For this review, take the finished solid that the model builds, in its own axes (mm). A direction names the side the tool comes from. Round coordinates to 2 decimals unless told otherwise and drop trailing zeros. Answer in a Markdown table with one row per item. Add a question column.
from build123d import *

# Parameters (mm, degrees)
BOSS_EXTRUDE1_START = -2
SKETCH2_R           = 33.5
BOSS_EXTRUDE1_DEPTH = 2
SKETCH3_W           = 10
SKETCH3_H           = 15
CUT_EXTRUDE1_DEPTH  = 2


with BuildPart() as part:
    # Sketch1 → Revolve1 (revolve)
    with BuildSketch(Plane.XY, mode=Mode.PRIVATE) as revolve1_sk:
        with BuildLine():
            Line((-33.5, 0), (-33.5, 29))
            Line((-33.5, 29), (-35, 29))
            Line((-35, 29), (-35, 34))
            add(Edge.make_bspline(
                [(-35, 34), (-35, 84.230477341), (-10.204077545, 129), (0, 129)],
                knots=[0, 0, 0, 0, 1, 1, 1, 1], degree=3))
            Line((0, 129), (0, 128))
            add(Edge.make_bspline(
                [(-33.998483451, 34.678650605), (-33.991581263, 36.224092512), (-33.93035746, 39.323038638), (-33.628011861, 45.449717858), (-32.930147658, 52.999936547), (-31.637237127, 61.816356904), (-29.381428766, 73.174794828), (-25.705936414, 86.483124789), (-20.381782509, 100.569855924), (-15.566274854, 110.353659681), (-11.721562917, 116.772432581), (-8.903323702, 120.821784375), (-6.216251644, 124.044106905), (-4.149084944, 125.985259834), (-2.652724981, 127.059465204), (-1.628060193, 127.620483156), (-0.879863894, 127.88514238), (-0.348657385, 127.984548618), (-0.119526866, 128), (0, 128)],
                knots=[0.004535476, 0.004535476, 0.004535476, 0.004535476, 0.035643742, 0.066752009, 0.128968542, 0.191185074, 0.253401607, 0.377834673, 0.502267738, 0.626700804, 0.688917336, 0.751133869, 0.813350402, 0.875566935, 0.906675201, 0.937783467, 0.968891734, 0.984445867, 1, 1, 1, 1], degree=3))
            Line((-33.998483451, 34.678650605), (-34, 33.678651755))
            Line((-34, 33.678651755), (-34, 30))
            Line((-34, 30), (-32.5, 30))
            Line((-32.5, 30), (-32.5, 0))
            Line((-32.5, 0), (-33.5, 0))
        make_face()
    revolve(revolve1_sk.sketch.rotate(Axis((0, 0, 0), (0, 1, 0)), 270), axis=Axis((0, 0, 0), (0, 1, 0)))

    # Sketch2 → Boss-Extrude1 (add)
    with BuildSketch(Plane.XZ.offset(BOSS_EXTRUDE1_START)):
        with Locations(Location((0, 0, 0), (0, 0, 270))):
            Circle(SKETCH2_R)
    extrude(amount=BOSS_EXTRUDE1_DEPTH)

    # Sketch3 → Cut-Extrude1 (cut)
    with BuildSketch(Plane.XZ):
        with Locations((7.5, 0)):
            Rectangle(SKETCH3_W, SKETCH3_H)
        with Locations((-7.5, 0)):
            Rectangle(SKETCH3_W, SKETCH3_H)
    extrude(amount=-CUT_EXTRUDE1_DEPTH, mode=Mode.SUBTRACT)


solid = part.part
Q1. Tool access review of faces 4 (the face through (-33.71, 31.81, 4.43)), 5 (the face through (34, 29, 0)): name each direction out of +Z, -Z, +X, -X, +Y, -Y from which nothing blocks a thin tool from reaching the whole face with its end or side.
Q2. Insertion check: pin 1 Ø1.5 at (x, z) = (20.5, -28) entering from -Y; pin 2 Ø0.6 at (y, z) = (1, -1) entering from -X; pin 3 Ø5 at (y, z) = (28, 5.5) entering from -X. Each pin has a flat end and moves straight along its axis. Give the tip position at first contact, or say it passes through.
Q3. To check wall thickness, follow probe 1 along X at (y, z) = (32.05, 0); probe 2 along X at (y, z) = (17, 0); probe 3 along Y at (x, z) = (-21, 5). State the ranges of each line that lie inside material, in increasing order.
Q4. Draft analysis for pull direction Z (two halves, no side actions). For faces 1 (the face through (0, 0, 0)), 2 (the face through (-9.76, 15.8, -31)), 3 (the face through (21, 32, 28)), state which applies: released by +Z, released by -Z, zero draft, split by the parting line, or undercut.
Answer sheet:
| question | item | result |
|---|---|---|
| 1 | face 4 | none |
| 1 | face 5 | -Y |
| 2 | pin 1 | stops at y = 29 |
| 2 | pin 2 | stops at x = -33.49 |
| 2 | pin 3 | stops at x = -34.85 |
| 3 | probe 1 | x = -35 to -34, 34 to 35 |
| 3 | probe 2 | x = -33.5 to -32.5, 32.5 to 33.5 |
| 3 | probe 3 | y = 0 to 2, 97.11 to 99.72 |
| 4 | face 1 | zero draft |
| 4 | face 2 | undercut |
| 4 | face 3 | split by the parting line |
